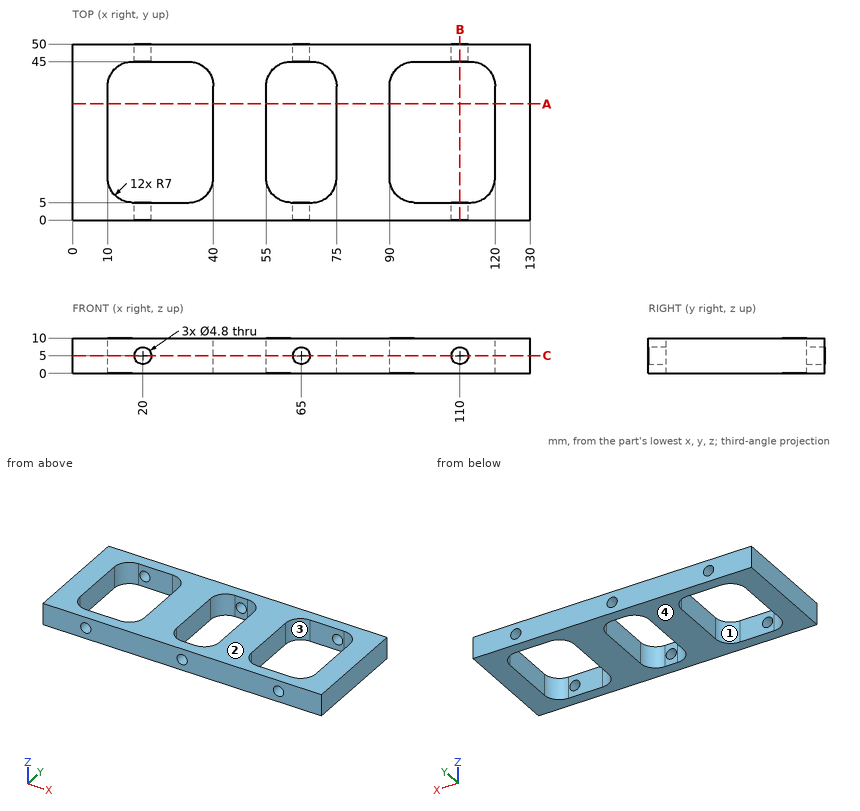
Here's the drawing with two shaded views (mm, measured from the low corner). I have some questions. A direction names the side the tool comes from. Give positions to 0.01 mm unless a question says otherwise; leave off trailing zeros. Loops run counter-clockwise (first coordinate to the right, second up) from the corner with the lowest first, then second, coordinate; pieces in that order, holes last. Notation, with made-up numbers: M -35.5,84.5 L -7.5,84.5 A21 cw -7.5,119.5 Z; hole C 42.25,24 d8. An arc over 180 degrees is marked long. Use one line per item in the form item = value. Start each with the question number.
(1) I want a section at C-C, the plane z = 5. State how many separate pieces and enclosed holes the cut face has, and give its area (3 significant figures).
(2) I want a section at A-A, the plane y = 33. Write out the boundary of the cut face in (x, z), and give its area (3 significant figures).
(3) I want a section at B-B, the plane x = 110. Write out the boundary of the cut face in (y, z), and give its area (3 significant figures).
(4) On a 3-axis mill with a long thin cutter (end or side, diameter ignored), from which of +Z, -Z, +X, -X, +Y, -Y can I reach the whole of each face in a straight line? I mean the marked faces 3 and 4. Say none if no direction works.
(5) Thinking about a two-plate mould opening in X: for the marked faces 1 and 2, which applies, released by +X, released by -X, zero draft, split by the parting line, or undercut?
(6) I'm going to push a flat-ended pin straight in: P1, Ø6, axis at x = 95.5, y = 40.5, coming from the +Z side. Where does the tip first touch, or does it pass through?
(7) Please list where these lines run through material, in increasing order: line 1 (X direction, y = 25, z = 6); line 2 (X direction, y = 2.95, z = 5); line 3 (Y direction, x = 25, z = 8).
Worked out:
q1.separate_pieces = 4
q1.enclosed_holes = 0
q1.area = 3,280 mm²
q2.outline = M 0,0 L 10,0 L 10,10 L 0,10 Z; M 40,0 L 55,0 L 55,10 L 40,10 Z; M 75,0 L 90,0 L 90,10 L 75,10 Z; M 120,0 L 130,0 L 130,10 L 120,10 Z
q2.area = 500 mm²
q3.outline = M 0,0 L 5,0 L 5,2.6 L 0,2.6 Z; M 0,7.4 L 5,7.4 L 5,10 L 0,10 Z; M 45,0 L 50,0 L 50,2.6 L 45,2.6 Z; M 45,7.4 L 50,7.4 L 50,10 L 45,10 Z
q3.area = 52.0 mm²
q4.face_3 = +Z, -Z
q4.face_4 = -Z, +X, -X, +Y, -Y
q5.face_1 = undercut
q5.face_2 = zero draft
q6.P1 = through
q7.line_1 = 0 to 10, 40 to 55, 75 to 90, 120 to 130
q7.line_2 = 0 to 17.6, 22.4 to 62.6, 67.4 to 107.6, 112.4 to 130
q7.line_3 = 0 to 5, 45 to 50
